Geometry: final body of the model. Coordinates: model frame, mm. A direction names the side the tool comes from. Give positions to 0.01 mm unless a question says otherwise; leave off trailing zeros. Write each loop counter-clockwise with the first axis right and the second up, starting at its lowest first coordinate (ties: lowest second). Pieces come first, ordered by that corner, then holes. Notation, with made-up numbers: (33.5, -9.5) -> (64.5, -9.5) arc R27 cw to (64.5, 11.5) -> close; hole circle Ø1 at (12.25, 14). An arc over 180 degrees is marked (long way). Answer as a JSON object with one key per item and string values.
from build123d import *

# Parameters (mm, degrees)
SKETCH007_W      = 229.65287
SKETCH007_H      = 196.321915
POCKET003_DEPTH  = 10
HOLE_D           = 3.1
HOLE_DEPTH       = 25
HOLE_CSINK_D     = 8
HOLE_CSINK_ANGLE = 90
SKETCH009_W      = 30
SKETCH009_H      = 2
POCKET004_DEPTH  = 30


with BuildPart() as bearing_outside:
    # Sketch003 → Revolution001 (revolve)
    with BuildSketch(Plane.XZ):
        with BuildLine():
            Line((27, 2), (27, 0))
            Line((27, 0), (50, 0))
            Line((50, 0), (50, 5))
            Line((50, 5), (16, 5))
            Line((16, 5), (16, 2))
            Line((16, 2), (16.918335, 2))
            ThreePointArc((19.081665, 2), (18, 2.9), (16.918335, 2))
            Line((19.081665, 2), (20, 2))
            Line((20, 2), (27, 2))
        make_face()
    revolve(axis=Axis((0, 0, 0), (0, 0, 1)))

    # Sketch007 (on Face6 of Revolution001) → Pocket003 (cut)
    with BuildSketch(Plane(origin=(0, 0, 5), x_dir=(-1, 0, 0), z_dir=(0, 0, 1))):
        with Locations((6.373165, -15.747734)):
            Rectangle(SKETCH007_W, SKETCH007_H)
        Polygon((30, 30), (30, -30), (-25, -30), (-25, -25), (-35, -25), (-35, 15), (-25, 15), (-25, 30), align=None, mode=Mode.SUBTRACT)
    extrude(amount=-POCKET003_DEPTH, mode=Mode.SUBTRACT)

    # Hole
    with Locations(Plane(origin=(0, 0, 5), x_dir=(-1, 0, 0), z_dir=(0, 0, 1))):
        with Locations((25, 25), (25, -25), (-30, -15), (-30, 5)):
            CounterSinkHole(HOLE_D / 2, HOLE_CSINK_D / 2, depth=HOLE_DEPTH, counter_sink_angle=HOLE_CSINK_ANGLE)

    # Sketch009 (on Face13 of Hole) → Pocket004 (cut)
    with BuildSketch(Plane(origin=(0, 30, 0), x_dir=(1, 0, 0), z_dir=(0, 1, 0))):
        with Locations((-9, -1)):
            Rectangle(SKETCH009_W, SKETCH009_H)
    extrude(amount=-POCKET004_DEPTH, mode=Mode.SUBTRACT)


with BuildPart() as part_mirroring:
    # Part__Mirroring: instance of bearing-outside
    add(bearing_outside.part.mirror(Plane(origin=(0, 0, 0), x_dir=(0, 1, 0), z_dir=(0, 0, 1))))


solid = part_mirroring.part
Q1. Material intervals for L1, parallel to Y at x = 30, z = -1.4; L2, parallel to X at y = 15, z = -0.6; L3, parallel to Y at x = -26, z = -3.2, sorted ascending. Write a range as from..to.
Values:
{"L1": "-15..-6.55, -3.45..13.45, 16.55..25", "L2": "-30..-24, 22.45..28.45, 31.55..35", "L3": "-30..-26.96, -23.04..23.04, 26.96..30"}
Q2. Cut plane A-A (z = -3.65). Return the cut outline in (x, y).
Values:
{"outline": "(-30, -30) -> (25, -30) -> (25, -15) -> (35, -15) -> (35, 25) -> (25, 25) -> (25, 30) -> (-30, 30) -> close; hole circle Ø5.3 at (-25, -25); hole circle Ø5.3 at (-25, 25); hole circle Ø32 at (0, 0); hole circle Ø5.3 at (30, -5); hole circle Ø5.3 at (30, 15)"}
Q3. Cut plane C-C (x = 30). Return the cut outline in (y, z).
Values:
{"outline": "(-15, -5) -> (-9, -5) -> (-6.55, -2.55) -> (-6.55, 0) -> (-15, 0) -> close; (-3.45, -2.55) -> (-1, -5) -> (11, -5) -> (13.45, -2.55) -> (13.45, 0) -> (-3.45, 0) -> close; (16.55, -2.55) -> (19, -5) -> (25, -5) -> (25, 0) -> (16.55, 0) -> close"}
Q4. Cut plane D-D (x = 0). Return the cut outline in (y, z).
Values:
{"outline": "(-30, -5) -> (-16, -5) -> (-16, -2) -> (-16.92, -2) arc R1.1 cw to (-19.08, -2) -> (-27, -2) -> (-27, 0) -> (-30, 0) -> close; (16, -5) -> (30, -5) -> (30, -2) -> (19.08, -2) arc R1.1 cw to (16.92, -2) -> (16, -2) -> close"}
Q5. Cut plane B-B (y = 0). Return the cut outline in (x, z).
Values:
{"outline": "(-30, -5) -> (-16, -5) -> (-16, -2) -> (-16.92, -2) arc R1.1 cw to (-19.08, -2) -> (-27, -2) -> (-27, 0) -> (-30, 0) -> close; (16, -5) -> (35, -5) -> (35, 0) -> (27, 0) -> (27, -2) -> (19.08, -2) arc R1.1 cw to (16.92, -2) -> (16, -2) -> close"}
Q6. Set-up query: faces 4 (the flat face through (-18, 8, -2)), 5 (the flat face through (6, 28, -1)), 6 (the flat face through (30, -15, -3)). Return all of +Z, -Z, +X, -X, +Y, -Y with unobstructed straight access to the full face (end or side cutting, diameter ignored); none if empty.
Values:
{"face 4": "+Z", "face 5": "+Z, +Y", "face 6": "+Z, -Z, +X, -Y"}
Q7. First-contact query: P1, Ø2, axis at y = 27.5, z = -1, coming from the +X side; P2, Ø4, axis at x = -25, y = -25, coming from the -Z side; P3, Ø1.5, axis at x = 29, z = -3, coming from the -Y side. Flat tips, straight axial feed; report the tip coordinate or a pass-through.
Values:
{"P1": "x = 25", "P2": "z = -3", "P3": "y = -15"}
Q8. Mould query, pull axis Y, two halves, no side actions, for faces 1 (the flat face through (30, 25, -3)), 2 (the cylindrical face through (31.478, 14.534, -1.257)), 3 (the flat face through (27, -4, 0)). Classes: pulls with the +Y half, pulls with the -Y half, needs draft (parallel to the pull), parting line crosses it, or undercut.
Values:
{"face 1": "pulls with the +Y half", "face 2": "undercut", "face 3": "needs draft"}
